Build history of the part. All positions in model axes, mm. A direction names the side the tool comes from. Give positions to 0.01 mm unless a question says otherwise; leave off trailing zeros. Order: outer loops, then holes, each group sorted by start corner. A loop starts at its lowest first (then second) coordinate and runs counter-clockwise, first axis right, second up. Notation, with made-up numbers: (37.5, -21) - (86.5, -21) arc R30 ccw to (86.5, 14) - close; hole circle Ø8 at (70.25, -28.75). An arc over 180 degrees is marked (long way). One line per item, written item: value.
```python
from build123d import *

# Parameters (mm, degrees)
F0_W     = 90
F0_H     = 160
F1_DEPTH = 88
F2_W     = 80
F2_H     = 9
F3_DEPTH = 12.5
F4_DEPTH = 50
F5_R     = 17.988747928
F6_DEPTH = 10
F7_R     = 15.1004844519
F8_DEPTH = 10
F9_R     = 4.99999


# Not quite as in the source:
# - a fillet or chamfer is up to 0.001 mm smaller than in the source, because OpenCascade refuses the exact size


with BuildPart() as f1:
    # F0 (on Top) → F1 (new body)
    with BuildSketch(Plane.XY):
        Rectangle(F0_W, F0_H)
    extrude(amount=F1_DEPTH)

    # F2 (on face) → F3 (cut, symmetric)
    with BuildSketch(Plane.XY.offset(88)):
        with Locations((0, 41.9618518679)):
            Rectangle(F2_W, F2_H)
    extrude(amount=F3_DEPTH, both=True, mode=Mode.SUBTRACT)

    # F4 (cut): a face of the model
    f4_faces = [f1.faces().sort_by_distance(p)[0] for p in [
        (0, 41.9618518679, 75.5),
    ]]
    extrude(f4_faces, amount=-F4_DEPTH, mode=Mode.SUBTRACT)

    # F5 (on face) → F6 (join)
    with BuildSketch(Plane.XZ.offset(80)):
        with Locations((0, 43)):
            Circle(F5_R)
    extrude(amount=F6_DEPTH)

    # F7 (on face) → F8 (cut)
    with BuildSketch(Plane.XZ.offset(90)):
        with Locations((0, 43)):
            Circle(F7_R)
    extrude(amount=-F8_DEPTH, mode=Mode.SUBTRACT)

    # F9 (radius 5 in the source; OpenCascade refuses exactly that, so slightly less here)
    f9_edges = [f1.edges().sort_by_distance(p)[0] for p in [
        (-45, 0, 88),
        (45, 0, 88),
        (45, 0, 0),
        (-45, 0, 0),
    ]]
    fillet(f9_edges, radius=F9_R)


solid = f1.part
```
(1) 3-axis set-ups, long thin cutter, end or side, ignore diameter. For faces 1 (the face through (-40, 42, 57)), 2 (the face through (-1, 1, 88)), 3 (the face through (-1, -80, 24)): which of +Z, -Z, +X, -X, +Y, -Y reach the whole face in a straight line?
Completed:
face 1: +Z
face 2: +Z, +X, -X, +Y, -Y
face 3: -Y
(2) Drill centre lines: line 1 (Y direction, x = 26.5, z = 82); line 2 (Z direction, x = 0, y = -82.5); line 3 (Y direction, x = 10.5, z = 28.5). Where is each one in solid material? Low to high.
Completed:
line 1: -80 to 37.46, 46.46 to 80
line 2: 25.01 to 27.9, 58.1 to 60.99
line 3: -90 to 37.46, 46.46 to 80
(3) Slice it at B-B, the plane x = 0. Give the cut face in (y, z), and give its area (3 significant figures).
Completed:
outline: (-90, 25.01) - (-80, 25.01) - (-80, 0) - (80, 0) - (80, 88) - (46.46, 88) - (46.46, 25.5) - (37.46, 25.5) - (37.46, 88) - (-80, 88) - (-80, 60.99) - (-90, 60.99) - (-90, 58.1) - (-80, 58.1) - (-80, 27.9) - (-90, 27.9) - close
area: 13,600 mm²
(4) Slice it at C-C, the plane z = 17. Give the cut face in (x, y), and give its area (3 significant figures).
Completed:
outline: (-45, -80) - (45, -80) - (45, 80) - (-45, 80) - close
area: 14,400 mm²
(5) Slice it at A-A, the plane z = 43. Give the cut face in (x, y), and give its area (3 significant figures).
Completed:
outline: (-45, -80) - (-17.99, -80) - (-17.99, -90) - (-15.1, -90) - (-15.1, -80) - (15.1, -80) - (15.1, -90) - (17.99, -90) - (17.99, -80) - (45, -80) - (45, 80) - (-45, 80) - close; hole (-40, 37.46) - (40, 37.46) - (40, 46.46) - (-40, 46.46) - close
area: 13,700 mm²
(6) Slice it at D-D, the plane x = 20.5. Give the cut face in (y, z), and give its area (3 significant figures).
Completed:
outline: (-80, 0) - (80, 0) - (80, 88) - (46.46, 88) - (46.46, 25.5) - (37.46, 25.5) - (37.46, 88) - (-80, 88) - close
area: 13,500 mm²
(7) Pin check, flat tips, straight feed: P1, Ø9, axis at x = -7.5, z = 48.5, coming from the -Y side; P2, Ø2.5, axis at x = -10.5, y = 41, coming from the +Z side. Stop position of each tip, or through.
Completed:
P1: y = -80
P2: z = 25.5
(8) Pull direction X, two halves, no side cores. Call faces 4 (the face through (-2.342, -84.93, 60.836)), 5 (the face through (-4, -90, 58)), 6 (the face through (40, 42, 57)): +X half, -X half, draft (parallel to the pull), parting line (faces both ways), or undercut.
Completed:
face 4: parting line
face 5: draft
face 6: undercut
